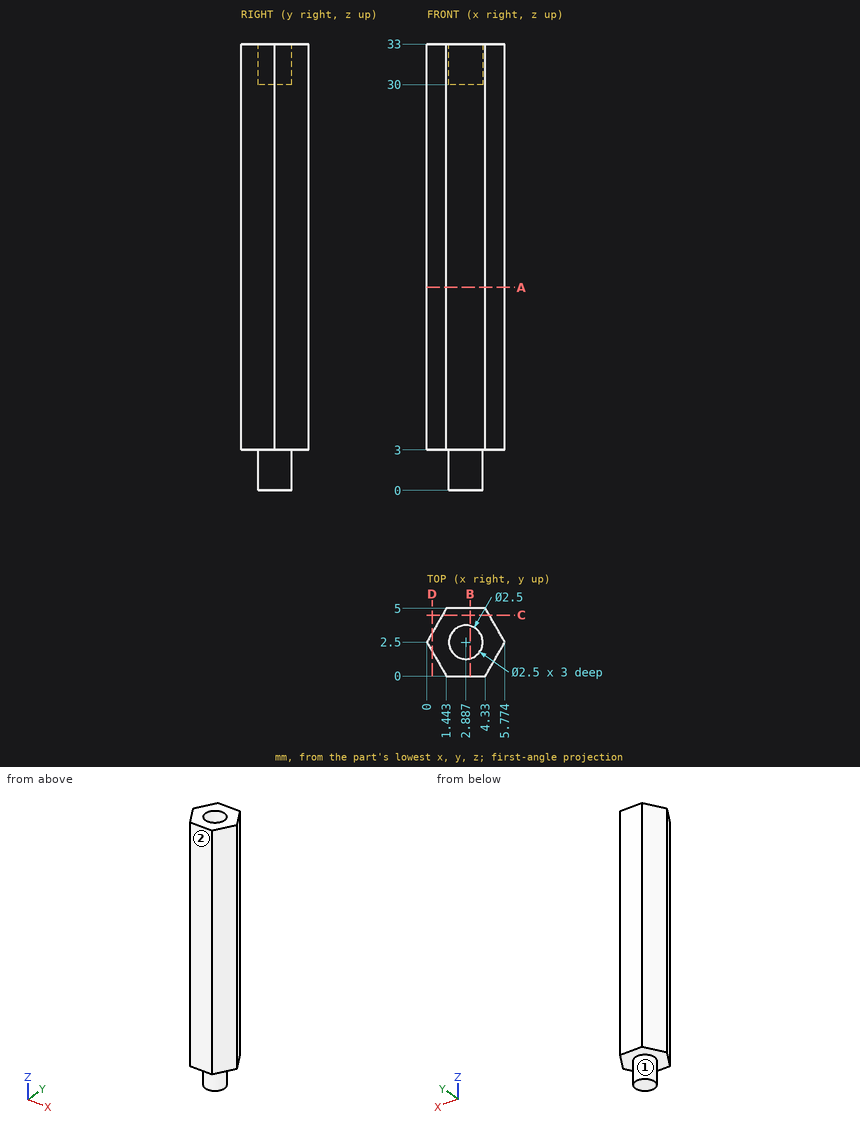
Geometry check sheet. Reference: drawing and pictorial views, mm from the part's lowest x, y, z. A direction names the side the tool comes from. Round coordinates to 2 decimals unless told otherwise and drop trailing zeros. Order: outer loops, then holes, each group sorted by start corner. A loop starts at its lowest first (then second) coordinate and runs counter-clockwise, first axis right, second up. Notation, with made-up numbers: (73.5, -27) - (98.5, -27) arc R34 ccw to (98.5, 5) - close; hole circle Ø1 at (-12.5, 78). An arc over 180 degrees is marked (long way). One line per question, with ' | ' between items. Start each with the question number.
(1) Sectioned sample at A-A on z = 15. Record the cut outline in (x, y).
(2) Thickness scan on L1, parallel to Z at x = 2.8, y = 2.15; L2, parallel to Y at x = 5.1, z = 27 (1 decimal); L3, parallel to X at y = 1.65, z = 28. Record the ranges inside material, lowest first. Write a range as [from, to].
(3) Sectioned sample at B-B on x = 3.2. Record the cut outline in (y, z), and give its area (3 significant figures).
(4) Depth check by flat-ended pin: pin 1 Ø1 at (y, z) = (3.5, 26) entering from -X. Enter the tip coordinate at first touch or a pass-through.
(5) Sectioned sample at C-C on y = 4.5. Record the cut outline in (x, z) (1 decimal).
(6) Sectioned sample at D-D on x = 0.4. Record the cut outline in (y, z).
(7) Access from +Z, -Z, +X, -X, +Y, -Y to the whole of each face (thin tool, end or side, straight path). Record for the marked faces 1 and 2.
Conclusion:
1) outline: (0, 2.5) - (1.44, 0) - (4.33, 0) - (5.77, 2.5) - (4.33, 5) - (1.44, 5) - close
2) L1: z = [0, 30] | L2: y = [1.3, 3.7] | L3: x = [0.49, 5.28]
3) outline: (0, 3) - (1.29, 3) - (1.29, 0) - (3.71, 0) - (3.71, 3) - (5, 3) - (5, 33) - (3.71, 33) - (3.71, 30) - (1.29, 30) - (1.29, 33) - (0, 33) - close | area: 150 mm2
4) pin 1: stops at x = 0.29
5) outline: (1.2, 3) - (4.6, 3) - (4.6, 33) - (1.2, 33) - close
6) outline: (1.81, 3) - (3.19, 3) - (3.19, 33) - (1.81, 33) - close
7) face 1: -Z | face 2: +Z, -Z, +X, -X, -Y
